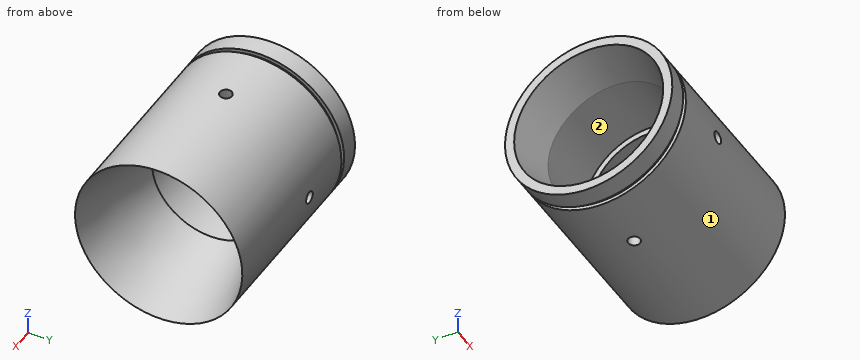
from build123d import *

# Parameters (mm, degrees)
SKETCH2_R          = 2.5
CUT_EXTRUDE1_DEPTH = 5
CIRPATTERN1_COUNT  = 4


with BuildPart() as part:
    # Sketch1 → Revolve1 (revolve)
    with BuildSketch(Plane.XY, mode=Mode.PRIVATE) as revolve1_sk:
        Polygon((11.626929507, 34.798), (19.723685425, 34.798), (19.723685425, 33.198), (21.723685425, 33.198), (21.723685425, 34.798), (95.442270017, 34.798), (56.73579947, 24.426632475), (56.73579947, 26.944570435), (29.496610327, 26.944570435), (11.626929507, 31.001470945), align=None)
    revolve(revolve1_sk.sketch.rotate(Axis((0, 0, 0), (1, 0, 0)), 90), axis=Axis((0, 0, 0), (1, 0, 0)))

    # Sketch2 → Cut-Extrude1 (cut)
    with BuildSketch(Plane(origin=(0, 34.798, 0), x_dir=(1, 0, 0), z_dir=(0, 1, 0))):
        with Locations(Location((45.442270017, 0, 0), (0, 0, 270))):
            Circle(SKETCH2_R)
    cut_extrude1 = extrude(amount=-CUT_EXTRUDE1_DEPTH, mode=Mode.SUBTRACT)

    # CirPattern1: Cut-Extrude1 ×4 about axis
    cirpattern1_axis = Axis((0, 0, 0), (1, 0, 0))
    for i in range(1, CIRPATTERN1_COUNT):
        add(cut_extrude1.rotate(cirpattern1_axis, i * 360 / CIRPATTERN1_COUNT), mode=Mode.SUBTRACT)


solid = part.part
CAD build for the part. Positions are in the model's coordinates, mm. Face numbers are marked on the shaded views. Coordinates: 2 decimals unless noted, no trailing zeros. Order: outer loops, then holes, each group sorted by start corner. A loop starts at its lowest first (then second) coordinate and runs counter-clockwise, first axis right, second up.
Item 1: Two-plate mould, pull along Y, no slides. Class the marked faces 1 and 2: +Y half, -Y half, draft (parallel to the pull), parting line (faces both ways), or undercut.
Check sheet entries:
face 1: parting line
face 2: undercut
Item 2: Pin check, flat tips, straight feed: pin 1 Ø4 at (x, z) = (46.5, 0.5) entering from -Y; pin 2 Ø3 at (x, z) = (45.44, 0) entering from +Y; pin 3 Ø1.5 at (x, y) = (45.5, -0.5) entering from -Z; pin 4 Ø2 at (x, y) = (48, 25.5) entering from -Z. Stop position of each tip, or through.
Check sheet entries:
pin 1: stops at y = -34.8
pin 2: stops at y = 29.8
pin 3: stops at z = -29.8
pin 4: stops at z = -24.71
Item 3: Band-saw the part on D-D on x = 24.5. List the corners of the cut face in (y, z), plus the area to 3 significant figures.
Check sheet entries:
outline: circle Ø69.6 at (0, 0); hole circle Ø56.16 at (0, 0)
area: 1,330 mm2
Item 4: Band-saw the part on A-A on y = 0. List the corners of the cut face in (x, z).
Check sheet entries:
outline: (11.63, -34.8) - (19.72, -34.8) - (19.72, -33.2) - (21.72, -33.2) - (21.72, -34.8) - (42.94, -34.8) - (42.94, -29.8) - (47.94, -29.8) - (47.94, -34.8) - (95.44, -34.8) - (56.74, -24.43) - (56.74, -26.94) - (29.5, -26.94) - (11.63, -31) - close; (11.63, 31) - (29.5, 26.94) - (56.74, 26.94) - (56.74, 24.43) - (95.44, 34.8) - (47.94, 34.8) - (47.94, 29.8) - (42.94, 29.8) - (42.94, 34.8) - (21.72, 34.8) - (21.72, 33.2) - (19.72, 33.2) - (19.72, 34.8) - (11.63, 34.8) - close
Item 5: Drill centre lines: L1, parallel to Y at x = 45.5, z = 0; L2, parallel to Z at x = 82.5, y = 6.5; L3, parallel to Y at x = 67.5, z = -10. Where is each one in solid material? Low to high.
Check sheet entries:
L1: y = -29.8 to -26.94, 26.94 to 29.8
L2: z = -34.19 to -30.65, 30.65 to 34.19
L3: y = -33.33 to -25.41, 25.41 to 33.33
Item 6: Band-saw the part on C-C on x = 62. List the corners of the cut face in (y, z), plus the area to 3 significant figures.
Check sheet entries:
outline: circle Ø69.6 at (0, 0); hole circle Ø51.67 at (0, 0)
area: 1,710 mm2
